Here's how the part is built. I have some questions about the finished solid (model axes, mm). Round coordinates to 2 decimals unless told otherwise and drop trailing zeros. Order: outer loops, then holes, each group sorted by start corner. A loop starts at its lowest first (then second) coordinate and runs counter-clockwise, first axis right, second up. Notation, with made-up numbers: (35, 23) -> (54, 23) arc R12 ccw to (54, 33) -> close; hole circle Ø11 at (11.5, 89). An arc over 180 degrees is marked (long way). Use a Markdown table: item, result. Add a question column.
from build123d import *

# Parameters (mm, degrees)
F1_DEPTH = 61.8998
F3_DEPTH = 92.806324
F4_DEPTH = 25.4


with BuildPart() as f1:
    # F0 (on Top) → F1 (new body)
    with BuildSketch(Plane.XY):
        with BuildLine():
            Line((-10.236888, 232.51189), (-0.534554, 12.141394))
            ThreePointArc((-0.534554, 12.141394), (3.372617, 3.524372), (12.153155, 0))
            Line((12.153155, 0), (70.396845, 0))
            ThreePointArc((70.396845, 0), (79.177383, 3.524372), (83.084554, 12.141394))
            Line((83.084554, 12.141394), (92.786888, 232.51189))
            ThreePointArc((92.786888, 232.51189), (87.518766, 246.520607), (73.755324, 252.3998))
            Line((73.755324, 252.3998), (8.794676, 252.3998))
            ThreePointArc((8.794676, 252.3998), (-4.968766, 246.520607), (-10.236888, 232.51189))
        make_face()
    extrude(amount=F1_DEPTH)

    # F2 (on Right) → F3 (cut, through all)
    with BuildSketch(Plane.YZ):
        Polygon((0, 61.8998), (252.3998, 57.15), (252.3998, 61.8998), align=None)
    extrude(amount=F3_DEPTH, mode=Mode.SUBTRACT)

    # F2 (on Right) → F4 (cut)
    with BuildSketch(Plane.YZ):
        Polygon((0, 61.8998), (252.3998, 57.15), (252.3998, 61.8998), align=None)
    extrude(amount=-F4_DEPTH, mode=Mode.SUBTRACT)


solid = f1.part
(1) I want a section at C-C on y = 145. List the corners of the cut face in (x, z) for me.
(2) I want a section at A-A on z = 53. List the corners of the cut face in (x, y) for me, and give its area (3 significant figures).
(3) I want a section at B-B on x = 20. List the corners of the cut face in (y, z) for me.
(4) Please list where these lines run through material, in increasing order: probe 1 along Z at (x, y) = (56, 235.5); probe 2 along Y at (x, z) = (12, 12); probe 3 along Y at (x, z) = (80.5, 28.5). Write a range as from..to.
(5) I'm going to push flat-ended pins straight in: P1, Ø10, axis at x = 7, z = 9, coming from the -Y side; P2, Ø3, axis at y = 110, z = 32, coming from the +X side; P3, Ø1.5, axis at x = 4, z = 10, coming from the -Y side. Where does each tip first touch, or does it pass through?
Output:
| question | item | result |
|---|---|---|
| 1 | outline | (-6.38, 0) -> (88.93, 0) -> (88.93, 59.17) -> (-6.38, 59.17) -> close |
| 2 | outline | (-10.24, 232.51) -> (-0.53, 12.14) arc R12.7 ccw to (12.15, 0) -> (70.4, 0) arc R12.7 ccw to (83.08, 12.14) -> (92.79, 232.51) arc R19.05 ccw to (73.76, 252.4) -> (8.79, 252.4) arc R19.05 ccw to start |
| 2 | area | 23,400 mm² |
| 3 | outline | (0, 0) -> (252.4, 0) -> (252.4, 57.15) -> (0, 61.9) -> close |
| 4 | probe 1 | 0..57.47 |
| 4 | probe 2 | 0..252.4 |
| 4 | probe 3 | 5..251.17 |
| 5 | P1 | y = 0 |
| 5 | P2 | x = 87.46 |
| 5 | P3 | y = 2.38 |
